Design review of the part built by this model. Coordinates are the model's own, in mm. Give positions to 0.01 mm unless a question says otherwise; leave off trailing zeros. Write each loop counter-clockwise with the first axis right and the second up, starting at its lowest first coordinate (ties: lowest second). Pieces come first, ordered by that corner, then holes. Notation, with made-up numbers: (50.25, -27.75) -> (70.25, -27.75) arc R27 ccw to (70.25, -8.75) -> close; hole circle Ø1 at (11.25, 6). An arc over 180 degrees is marked (long way). Use CSV: the item, a comma, the result in double quotes.
```python
from build123d import *

# Parameters (mm, degrees)
SKETCH1_R           = 8.75
SKETCH1_W           = 90
SKETCH1_H           = 17.5
BOSS_EXTRUDE1_DEPTH = 2.5
SKETCH2_R           = 2.5
CUT_EXTRUDE1_DEPTH  = 1007.034914901


with BuildPart() as part:
    # Sketch1 → Boss-Extrude1 (new body)
    with BuildSketch(Plane(origin=(2.5, 0, 0), x_dir=(0, 0, -1), z_dir=(1, 0, 0))):
        with BuildLine():
            Line((1000, 0), (1000, 100))
            ThreePointArc((1000, 100), (997.071067812, 107.071067812), (990, 110))
            Line((990, 110), (10, 110))
            ThreePointArc((10, 110), (2.928932188, 107.071067812), (0, 100))
            Line((0, 100), (0, 0))
            Line((0, 0), (1000, 0))
        make_face()
        with Locations(Location((136.5, 75, 0), (0, 0, 180))):
            Circle(SKETCH1_R, mode=Mode.SUBTRACT)
        with Locations(Location((186.5, 75, 0), (0, 0, 180))):
            Circle(SKETCH1_R, mode=Mode.SUBTRACT)
        with Locations(Location((256.5, 75, 0), (0, 0, 180))):
            Circle(SKETCH1_R, mode=Mode.SUBTRACT)
        with Locations(Location((326.5, 75, 0), (0, 0, 180))):
            Circle(SKETCH1_R, mode=Mode.SUBTRACT)
        with Locations(Location((396.5, 75, 0), (0, 0, 180))):
            Circle(SKETCH1_R, mode=Mode.SUBTRACT)
        with Locations(Location((466.5, 75, 0), (0, 0, 180))):
            Circle(SKETCH1_R, mode=Mode.SUBTRACT)
        with Locations(Location((536.5, 75, 0), (0, 0, 180))):
            Circle(SKETCH1_R, mode=Mode.SUBTRACT)
        with Locations(Location((606.5, 75, 0), (0, 0, 180))):
            Circle(SKETCH1_R, mode=Mode.SUBTRACT)
        with Locations(Location((676.5, 75, 0), (0, 0, 180))):
            Circle(SKETCH1_R, mode=Mode.SUBTRACT)
        with Locations(Location((746.5, 75, 0), (0, 0, 180))):
            Circle(SKETCH1_R, mode=Mode.SUBTRACT)
        with Locations(Location((816.5, 75, 0), (0, 0, 180))):
            Circle(SKETCH1_R, mode=Mode.SUBTRACT)
        with Locations(Location((886.5, 75, 0), (0, 0, 180))):
            Circle(SKETCH1_R, mode=Mode.SUBTRACT)
        with Locations(Location((956.5, 75, 0), (0, 0, 180))):
            Circle(SKETCH1_R, mode=Mode.SUBTRACT)
        with Locations((55, 75)):
            Rectangle(SKETCH1_W, SKETCH1_H, mode=Mode.SUBTRACT)
    extrude(amount=-BOSS_EXTRUDE1_DEPTH)

    # Sketch2 → Cut-Extrude1 (cut, through all)
    with BuildSketch(Plane(origin=(2.5, 0, 0), x_dir=(0, 0, -1), z_dir=(1, 0, 0))):
        with Locations((500, 100)):
            Circle(SKETCH2_R)
        with Locations((20, 100)):
            Circle(SKETCH2_R)
        with Locations((980, 100)):
            Circle(SKETCH2_R)
        with Locations((980, 30)):
            Circle(SKETCH2_R)
        with Locations((500, 30)):
            Circle(SKETCH2_R)
        with Locations((20, 30)):
            Circle(SKETCH2_R)
        with Locations((260, 100)):
            Circle(SKETCH2_R)
        with Locations((260, 30)):
            Circle(SKETCH2_R)
        with Locations((740, 100)):
            Circle(SKETCH2_R)
        with Locations((740, 30)):
            Circle(SKETCH2_R)
    extrude(amount=-CUT_EXTRUDE1_DEPTH, mode=Mode.SUBTRACT)


solid = part.part
```
(1) Take a section at B-B (x = 1.75). State how many separate pieces and enclosed holes the cut face has, then the cut area to 3 significant figures.
Established:
separate pieces,"1"
enclosed holes,"24"
area,"105,000 mm2"
(2) For line 1 along Z through (x, y) = (1.9, 98.5); line 2 along Y through (x, z) = (1.7, -536.5), list the stretches that pass through material, from the lowest coordinate up. Write a range as [from, to].
Established:
line 1,"z = [-1000, -982], [-978, -742], [-738, -502], [-498, -262], [-258, -22], [-18, 0]"
line 2,"y = [0, 66.25], [83.75, 110]"
(3) Mouldability with a two-part tool opening along Y and no side actions: class faces 1 (the face through (1.268, 72.372, -388.154)), 2 (the face through (0, 56, -493)) as +Y half, -Y half, draft (parallel to the pull), parting line (faces both ways), or undercut.
Established:
face 1,"undercut"
face 2,"draft"
(4) Take a section at A-A (z = -466.5). Write out the cut boundary in (x, y), then the cut area to 3 significant figures.
Established:
outline,"(0, 0) -> (2.5, 0) -> (2.5, 66.25) -> (0, 66.25) -> close; (0, 83.75) -> (2.5, 83.75) -> (2.5, 110) -> (0, 110) -> close"
area,"231 mm2"
(5) Clearance check with a flat-ended pin moving along its axis: pin 1 (8 mm diameter, centred on y = 72, z = -183.5, fed in from -X). State where the tip first meets the part, or that it passes through.
Established:
pin 1,"passes through"
